The model under review builds one solid part; all positions refer to its coordinate system, in mm. A direction names the side the tool comes from. Coordinates: 2 decimals unless noted, no trailing zeros. Loops run counter-clockwise (first coordinate to the right, second up) from the corner with the lowest first, then second, coordinate; pieces in that order, holes last. Notation, with made-up numbers: M 59.5,77 L 86.5,77 A7 ccw 86.5,84 Z; hole C -34,68.5 d3. An arc over 180 degrees is marked long. Write item = value, one per line. Start each with the question number.
Q1. We need section A-A on x = 0. Give the boundary of the cut face in (y, z) (1 decimal).
Q2. Clearance check with flat-ended pins moving along their axes: pin 1 Ø8 at (x, z) = (-2, 6) entering from -Y; pin 2 Ø2.5 at (y, z) = (-39.5, -0.5) entering from +X; pin 3 Ø1.6 at (x, y) = (8.5, -39.5) entering from +Z. State where each tip first meets the part, or that it passes through.
Q3. Wall thickness on probe 1 along Z at (x, y) = (-0.25, -11.5); probe 2 along Y at (x, z) = (-3.25, 0.5); probe 3 along X at (y, z) = (-28, 0) (1 decimal): over which ranges is each line inside the solid? List them lowest first.
Q4. For faces 4 (the face through (-3.23, 37.78, 5.54)), 5 (the face through (-0.1, -19.698, -3.4)), 6 (the face through (6.35, -40, 0)), list the 3-axis set-ups (+Z, -Z, +X, -X, +Y, -Y) from which the entire face can be reached by the end or side of a thin tool; tool diameter is ignored.
Q5. Mouldability with a two-part tool opening along Z and no side actions: class faces 1 (the face through (-9.444, -10.374, 1.24)), 2 (the face through (8, -33.286, 0)), 3 (the face through (-7, 38.1, 1)) as released by +Z, released by -Z, zero draft, split by the parting line, or undercut.
from build123d import *

# Parameters (mm, degrees)
BOSS_EXTRUDE1_REACH = 81.121
SENSOR_R            = 6.35
CHAMFER1_SIZE       = 0.635
FILLET3_R           = 0.508
SKETCH4_R           = 4.445
CUT_EXTRUDE1_DEPTH  = 2.54
CUT_EXTRUDE2_DEPTH  = 3.175
CUT_EXTRUDE8_REACH  = 117.091
CIRPATTERN1_COUNT   = 6


with BuildPart() as part:
    # Sketch1 → mainBody (revolve)
    with BuildSketch(Plane(origin=(0, 0, 0), x_dir=(0, 0, -1), z_dir=(1, 0, 0)), mode=Mode.PRIVATE) as mainbody_sk:
        Polygon((-6.096, 38.1), (-6.096, 8.705990249), (0, 0), (0, -76.2), (-9.525, -59.702216058), (-9.525, 38.1), align=None)
    revolve(mainbody_sk.sketch.rotate(Axis((0, 0, 0), (0, 1, 0)), 180), axis=Axis((0, 0, 0), (0, 1, 0)))

    # sensor → Boss-Extrude1 (add, up to next)
    with BuildSketch(Plane(origin=(9.525, 0, 0), x_dir=(0, 0, -1), z_dir=(1, 0, 0)), mode=Mode.PRIVATE) as boss_extrude1_sk1:
        with Locations((0, -50.812216058)):
            Circle(SENSOR_R)
    boss_extrude1_tool1 = extrude(boss_extrude1_sk1.sketch, amount=-BOSS_EXTRUDE1_REACH, mode=Mode.PRIVATE) - part.part
    add(boss_extrude1_tool1.solids().sort_by_distance((9.525, -50.812216, 0))[0])
    add(boss_extrude1_tool1.solids().sort_by_distance((9.525, -50.812216, 0))[1])

    # Chamfer1
    chamfer1_edges = [part.edges().sort_by_distance(p)[0] for p in [
        (0, 38.1, 6.096),
    ]]
    chamfer(chamfer1_edges, length=CHAMFER1_SIZE)

    # Fillet3
    fillet3_edges = [part.edges().sort_by_distance(p)[0] for p in [
        (0, 38.1, 9.525),
    ]]
    fillet(fillet3_edges, radius=FILLET3_R)

    # Sketch4 → Cut-Extrude1 (cut)
    with BuildSketch(Plane(origin=(9.525, 0, 0), x_dir=(0, 0, -1), z_dir=(1, 0, 0))):
        with Locations((0, -50.812216058)):
            Circle(SKETCH4_R)
    extrude(amount=-CUT_EXTRUDE1_DEPTH, mode=Mode.SUBTRACT)

    # Sketch5 → Cut-Extrude2 (cut)
    with BuildSketch(Plane(origin=(9.525, 0, 0), x_dir=(0, 0, -1), z_dir=(1, 0, 0))):
        with BuildLine():
            Line((-1.5875, -33.286216058), (1.5875, -33.286216058))
            Line((1.5875, -33.286216058), (1.5875, -45.532735353))
            ThreePointArc((1.5875, -45.532735353), (0, -47.637216058), (-1.5875, -45.532735353))
            Line((-1.5875, -45.532735353), (-1.5875, -33.286216058))
        make_face()
    extrude(amount=-CUT_EXTRUDE2_DEPTH, mode=Mode.SUBTRACT)

    # Cut-Extrude8: up to this cone (the profile starts inside it)
    cut_extrude8_end = Plane(origin=(0, 38.1, 0), z_dir=(0, 1, 0)).offset(-38.099999) * Cone(1e-06, 127.696083561, 182.368906206, align=(Align.CENTER, Align.CENTER, Align.MIN), mode=Mode.PRIVATE)
    # Sketch13 → Cut-Extrude8 (cut, up to the surface)
    with BuildSketch(Plane(origin=(0, 38.1, 0), x_dir=(1, 0, 0), z_dir=(0, 1, 0)), mode=Mode.PRIVATE) as cut_extrude8_sk1:
        Polygon((-1.27, 8.001), (1.27, 8.001), (2.27589157, 2.296305428), (-2.27589157, 2.296305428), align=None)
    cut_extrude8_tool1 = extrude(cut_extrude8_sk1.sketch, amount=-CUT_EXTRUDE8_REACH, mode=Mode.PRIVATE) & cut_extrude8_end
    cut_extrude8 = cut_extrude8_tool1.solids().sort_by_distance((0, 38.1, -4.878937))[0]
    add(cut_extrude8, mode=Mode.SUBTRACT)

    # CirPattern1: Cut-Extrude8 ×6 about axis
    cirpattern1_axis = Axis((0, 0, 0), (0, 1, 0))
    for i in range(1, CIRPATTERN1_COUNT):
        add(cut_extrude8.rotate(cirpattern1_axis, i * 360 / CIRPATTERN1_COUNT), mode=Mode.SUBTRACT)

    # Sketch14 → Cut-Revolve4 (revolve, cut)
    with BuildSketch(Plane.XY, mode=Mode.PRIVATE) as cut_revolve4_sk:
        Polygon((0, -3.81), (7.9375, -3.81), (7.9375, -19.6977), (3.175, -19.6977), (3.175, -22.7457), (7.9375, -22.7457), (7.9375, -32.2707), (0, -32.2707), align=None)
    revolve(cut_revolve4_sk.sketch.rotate(Axis((0, 0, 0), (0, 1, 0)), 90), axis=Axis((0, 0, 0), (0, 1, 0)), mode=Mode.SUBTRACT)


solid = part.part
Returned:
q1.outline = M -76.2,0 L -59.7,-9.5 L 37.6,-9.5 A0.5 ccw 38.1,-9 L 38.1,-8 L 11.4,-8 L 0,0 L 11.4,8 L 38.1,8 L 38.1,9 A0.5 ccw 37.6,9.5 L -59.7,9.5 Z; hole M -32.3,-7.9 L -22.7,-7.9 L -22.7,-3.2 L -19.7,-3.2 L -19.7,-7.9 L -3.8,-7.9 L -3.8,7.9 L -19.7,7.9 L -19.7,3.2 L -22.7,3.2 L -22.7,7.9 L -32.3,7.9 Z
q2.pin_1 = -72.17
q2.pin_2 = 9.39
q2.pin_3 = 5.61
q3.probe_1 = -9.52 to -7.93, 7.93 to 9.52
q3.probe_2 = -70.5 to -32.27, -22.75 to -19.7, -3.81 to 4.7
q3.probe_3 = -9.5 to -7.9, 7.9 to 9.5
q4.face_4 = +Y
q4.face_5 = none
q4.face_6 = +X
q5.face_1 = split by the parting line
q5.face_2 = undercut
q5.face_3 = zero draft
